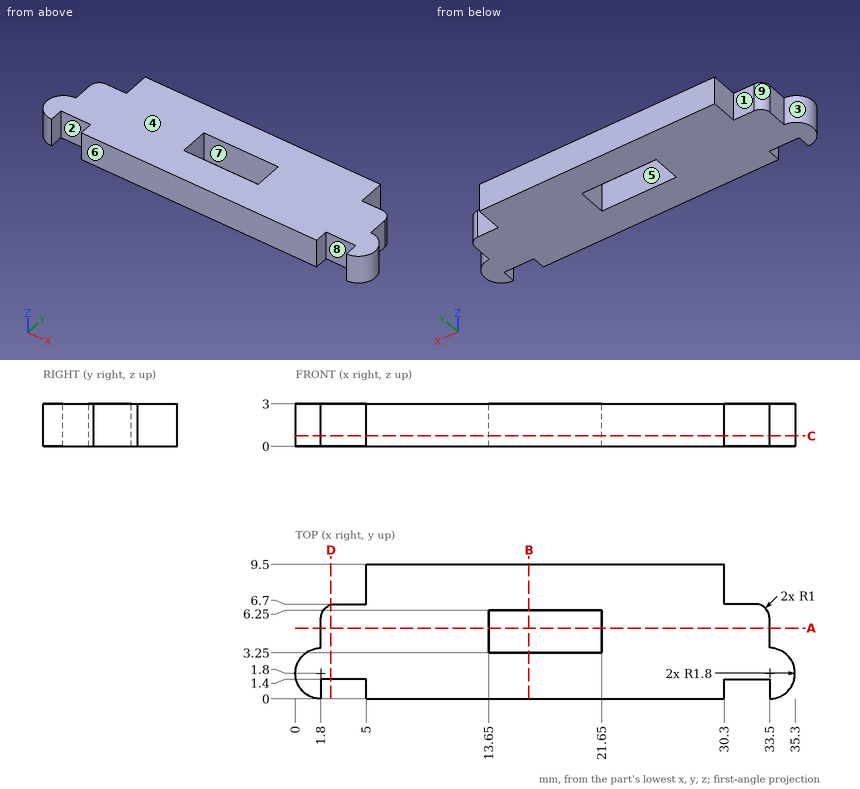
Can you work these out from the drawing? Everything is in mm from the part's minimum corner. A direction names the side the tool comes from. Round coordinates to 2 decimals unless told otherwise and drop trailing zeros. Loops run counter-clockwise (first coordinate to the right, second up) from the corner with the lowest first, then second, coordinate; pieces in that order, holes last. Notation, with made-up numbers: (41.25, -18.75) - (48.25, -18.75) arc R26 ccw to (48.25, 3.25) - close; hole circle Ø5 at (-13.5, 38). An arc over 180 degrees is marked (long way). Answer in a Markdown table with one row per item. Add a question column.
Q1. I want a section at A-A on y = 5. List the corners of the cut face in (x, z) for me.
Q2. Which directions (+Z, -Z, +X, -X, +Y, -Y) give clear straight access to the entire face, cutting with the end or side of a thin tool? Please do the marked faces 1, 2, 3, 4 and 5.
Q3. For pin 1 Ø1.4 at (y, z) = (7.5, 2) entering from +X; pin 2 Ø0.6 at (y, z) = (5, 1) entering from -X; pin 3 Ø0.6 at (y, z) = (4.5, 1.5) entering from +X, each with a flat end and sliding along its axis, tell me the tip position at first contact or that it passes through.
Q4. I want a section at D-D on x = 2.5. List the corners of the cut face in (y, z) for me.
Q5. I want a section at C-C on z = 0.75. List the corners of the cut face in (x, y) for me.
Q6. I need wall thicknesses on L1, parallel to X at y = 4.5, z = 1.2; L2, parallel to Y at x = 21, z = 0.65; L3, parallel to X at y = 0.75, z = 1. Which ranges of each line are inside material? Lowest first, please.
Q7. I want a section at B-B on x = 16.5. List the corners of the cut face in (y, z) for me, and give its area (3 significant figures).
Q8. We'd pull the mould along X, two halves only. Please class the marked faces 6, 7, 8 and 9: pulls with the +X half, pulls with the -X half, needs draft (parallel to the pull), parting line crosses it, or undercut.
A:
| question | item | result |
|---|---|---|
| 1 | outline | (1.8, 0) - (13.65, 0) - (13.65, 3) - (1.8, 3) - close; (21.65, 0) - (33.5, 0) - (33.5, 3) - (21.65, 3) - close |
| 2 | face 1 | +Z, -Z, -X, +Y |
| 2 | face 2 | +Z, -Z, -Y |
| 2 | face 3 | +Z, -Z, -X |
| 2 | face 4 | +Z, +X, -X, +Y, -Y |
| 2 | face 5 | +Z, -Z |
| 3 | pin 1 | x = 30.3 |
| 3 | pin 2 | x = 1.8 |
| 3 | pin 3 | x = 33.5 |
| 4 | outline | (1.4, 0) - (6.65, 0) - (6.65, 3) - (1.4, 3) - close |
| 5 | outline | (1.8, 0) - (1.8, 1.4) - (5, 1.4) - (5, 0) - (30.3, 0) - (30.3, 1.4) - (33.5, 1.4) - (33.5, 0) arc R1.8 ccw to (33.5, 3.6) - (33.5, 5.7) arc R1 ccw to (32.5, 6.7) - (30.3, 6.7) - (30.3, 9.5) - (5, 9.5) - (5, 6.7) - (2.8, 6.7) arc R1 ccw to (1.8, 5.7) - (1.8, 3.6) arc R1.8 ccw to start; hole (13.65, 3.25) - (21.65, 3.25) - (21.65, 6.25) - (13.65, 6.25) - close |
| 6 | L1 | 1.8 to 13.65, 21.65 to 33.5 |
| 6 | L2 | 0 to 3.25, 6.25 to 9.5 |
| 6 | L3 | 0.34 to 1.8, 5 to 30.3, 33.5 to 34.96 |
| 7 | outline | (0, 0) - (3.25, 0) - (3.25, 3) - (0, 3) - close; (6.25, 0) - (9.5, 0) - (9.5, 3) - (6.25, 3) - close |
| 7 | area | 19.5 mm^2 |
| 8 | face 6 | needs draft |
| 8 | face 7 | undercut |
| 8 | face 8 | undercut |
| 8 | face 9 | pulls with the -X half |
